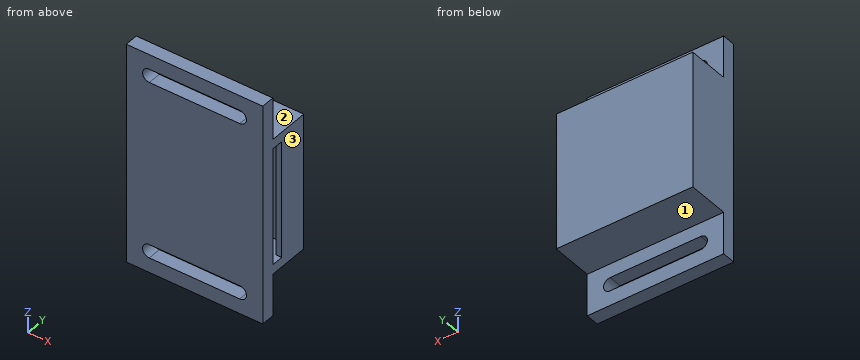
Autodesk Inventor part; units mm, degrees
ref_plane "YZ Plane" through (0, 0, 0) normal (1, 0, 0) x (0, 1, 0)
ref_plane "XZ Plane" through (0, 0, 0) normal (0, 1, 0) x (-1, 0, 0)
ref_plane "XY Plane" through (0, 0, 0) normal (0, 0, 1) x (1, 0, 0)
sketch "Sketch1" plane through (0, 0, 0) normal (0, 1, 0) x (-1, 0, 0)
  line L0 (15.25, -24.65) -> (-15.25, -24.65)
  line L1 (-15.25, -24.65) -> (-15.25, 24.65)
  line L2 (-15.25, 24.65) -> (15.25, 24.65)
  line L3 (15.25, 24.65) -> (15.25, -24.65)
  line L4 (15.25, -24.65) -> (-15.25, 24.65) construction
  line L5 (-15.25, -24.65) -> (15.25, 24.65) construction
  circle A0 centre (10.1, 19.85) radius 1.5
  circle A1 centre (-10.1, 19.85) radius 1.5
  line L6 (10.1, 21.35) -> (-10.1, 21.35)
  circle A2 centre (10.1, -19.85) radius 1.5
  circle A3 centre (-10.1, -19.85) radius 1.5
  line L7 (10.1, -21.35) -> (-10.1, -21.35)
  line L8 (21.35, 0) -> (-21.35, 0) construction
  line L9 (10.1, -18.35) -> (-10.1, -18.35)
  line L10 (10.1, 18.35) -> (-10.1, 18.35)
  line L11 (15.25, -15.25) -> (-15.25, -15.25)
  line L12 (-15.25, -15.25) -> (-15.25, 15.25)
  line L13 (-15.25, 15.25) -> (15.25, 15.25)
  line L14 (15.25, 15.25) -> (15.25, -15.25)
  line L15 (15.25, -15.25) -> (-15.25, 15.25) construction
  line L16 (-15.25, -15.25) -> (15.25, 15.25) construction
  line L17 (0, -34.51) -> (0, 34.51)
  point P0 (0, 0)
  dimension "d11" = 49.3
  dimension "d12" = 30.5
  dimension "d13" = 23.2
  dimension "d14" = 3
  dimension "d15" = 3.3
  dimension "d16" = 30.5
extrude "Extrusion1" add sketch "Sketch1" along normal blind 3 contours L0 L17 L7 A2 L9 L11 L3 | L0 L1 L11 L17 L9 A3 L7 | L11 L17 L13 L3 | L13 L17 L10 A0 L6 L2 L3 | L11 L1 L13 L17 | L13 L1 L2 L17 L6 A1 L10
extrude "Extrusion2" add sketch "Sketch1" along normal blind 12.3 contours L11 L17 L13 L3 | L11 L1 L13 L17
sketch "Sketch2" plane through (0, 12.3, 0) normal (0, 1, 0) x (1, 0, 0)
  line L0 (12.9324, 13.1) -> (-12.9324, 13.1)
  line L1 (-12.9324, 13.1) -> (-12.9324, -13.1)
  line L2 (-12.9324, -13.1) -> (12.9324, -13.1)
  line L3 (12.9324, -13.1) -> (12.9324, 13.1)
  line L4 (12.9324, 13.1) -> (-12.9324, -13.1) construction
  line L5 (-12.9324, 13.1) -> (12.9324, -13.1) construction
  point P0 (0, 0)
  dimension "d21" = 26.2
extrude "Extrusion3" cut sketch "Sketch2" against normal blind 9.3
sketch "Sketch3" plane through (12.9324, 12.3, -13.1) normal (-1, 0, 0) x (0, 0, 1)
  line L0 (26.2, 0) -> (26.2, -9.3)
  line L1 (26.2, -9.3) -> (0, -9.3)
  line L2 (0, 0) -> (0, -9.3)
  line L3 (-2.15, 0) -> (28.35, 0)
  line L4 (0, 0) -> (26.2, 0)
  line L5 (26.2, 0) -> (0, 0)
  line L6 (0, 0) -> (0, -9.3)
  line L7 (0, -9.3) -> (26.2, -9.3)
  line L8 (26.2, -9.3) -> (26.2, 0)
  point P0 (13.1, -12.3)
extrude "Extrusion4" cut sketch "Sketch3" against normal through all
sketch "Sketch6" plane through (0, 12.3, 0) normal (0, 1, 0) x (1, 0, 0)
  line L0 (-15.25, 15.25) -> (-15.25, -15.25)
  line L1 (15.25, 15.25) -> (15.25, 24.65)
  line L2 (-15.25, -15.25) -> (15.25, -15.25)
  line L3 (15.25, -15.25) -> (15.25, 15.25)
  line L4 (15.25, 15.25) -> (-15.25, 15.25)
  line L5 (-15.25, 15.25) -> (-15.25, -15.25)
  point P0 (0, 0)
extrude "Extrusion5" add sketch "Sketch6" against normal blind 3
sketch "Sketch7" plane through (0, 9.3, 0) normal (0, -1, 0) x (1, 0, 0)
  line L0 (15.25, 15.25) -> (15.25, -15.25)
  line L1 (-15.25, 15.25) -> (15.25, 15.25)
  line L2 (15.25, -15.25) -> (13.95, -15.25)
  line L3 (13.95, -15.25) -> (13.95, 15.25)
  line L4 (13.95, 15.25) -> (15.25, 15.25)
  line L5 (15.25, 15.25) -> (15.25, -15.25)
  line L6 (-15.25, -24.65) -> (-15.25, 24.65)
  point P0 (0, 0)
  dimension "d29" = 29.2
extrude "Extrusion6" add sketch "Sketch7" along normal blind 3.6
equation "\"d11\" = length"
equation "\"d12\" = width"
equation "\"d13\" = opening_length"
equation "\"d14\" = opening_width"
equation "\"d15\" = opening_distance_to_edge"
equation "\"d16\" = camera_box_width"
equation "\"d17\" = thickness"
equation "\"d19\" = height"
equation "\"d21\" = inside_width"
equation "\"d22\" = height - thickness"
equation "\"d26\" = thickness"
equation "\"d29\" = inside_width + thickness"
equation "\"d30\" = 1.2 * thickness"
equation "\"width\" = 30.5"
equation "\"length\" = 49.3"
equation "\"opening_width\" = 3"
equation "\"opening_length\" = 23.2"
equation "\"opening_distance_to_edge\" = 3.3"
equation "\"camera_box_width\" = 30.5"
equation "\"thickness\" = 3"
equation "\"inside_width\" = 26.2"
equation "\"height\" = 12.3"
properties part number "bottom" material "SAN Plastic"
The model under review builds one solid part; all positions refer to its coordinate system, in mm. Face numbers are marked on the shaded views. A direction names the side the tool comes from. Coordinates: 2 decimals unless noted, no trailing zeros. Write each loop counter-clockwise with the first axis right and the second up, starting at its lowest first coordinate (ties: lowest second). Pieces come first, ordered by that corner, then holes. Notation, with made-up numbers: (29.25, -23.75) -> (45.25, -23.75) arc R12 ccw to (45.25, -12.75) -> close; hole circle Ø9 at (76, 53). An arc over 180 degrees is marked (long way). Answer in a Markdown table with one row per item.
1. We need section C-C, the plane z = -7. State the section outline as (x, y) points.
Answers below:
| item | result |
|---|---|
| outline | (-15.25, 0) -> (15.25, 0) -> (15.25, 3) -> (-12.93, 3) -> (-12.93, 9.3) -> (13.95, 9.3) -> (13.95, 5.7) -> (15.25, 5.7) -> (15.25, 12.3) -> (-15.25, 12.3) -> close |
2. We need section A-A, the plane x = 3. State the section outline as (y, z) points, and give its area (3 significant figures).
Answers below:
| item | result |
|---|---|
| outline | (0, -24.65) -> (3, -24.65) -> (3, -21.35) -> (0, -21.35) -> close; (0, -18.35) -> (3, -18.35) -> (3, -15.25) -> (12.3, -15.25) -> (12.3, 15.25) -> (3, 15.25) -> (3, 18.35) -> (0, 18.35) -> close; (0, 21.35) -> (3, 21.35) -> (3, 24.65) -> (0, 24.65) -> close; hole (3, -13.1) -> (9.3, -13.1) -> (9.3, 13.1) -> (3, 13.1) -> close |
| area | 248 mm^2 |
3. We need section B-B, the plane y = 4. State the section outline as (x, z) points, and give its area (3 significant figures).
Answers below:
| item | result |
|---|---|
| outline | (-15.25, -15.25) -> (15.25, -15.25) -> (15.25, -13.1) -> (-12.93, -13.1) -> (-12.93, 13.1) -> (15.25, 13.1) -> (15.25, 15.25) -> (-15.25, 15.25) -> close |
| area | 192 mm^2 |
4. For the marked faces 1, 2 and 3, list the 3-axis set-ups (+Z, -Z, +X, -X, +Y, -Y) from which the entire face can be reached by the end or side of a thin tool; tool diameter is ignored.
Answers below:
| item | result |
|---|---|
| face 1 | -Z, +X, -X, +Y |
| face 2 | +Z, +X, -X, +Y |
| face 3 | +Z, -Z, +X, +Y, -Y |
5. Wall thickness on probe 1 along Z at (x, y) = (-7.5, 2.25); probe 2 along Y at (x, z) = (9, 2); probe 3 along Z at (x, y) = (6, 4): over which ranges is each line inside the solid? List them lowest first. Write a range as [from, to].
Answers below:
| item | result |
|---|---|
| probe 1 | z = [-24.65, -21.35], [-18.35, 18.35], [21.35, 24.65] |
| probe 2 | y = [0, 3], [9.3, 12.3] |
| probe 3 | z = [-15.25, -13.1], [13.1, 15.25] |
6. We need section D-D, the plane y = 8. State the section outline as (x, z) points, and give its area (3 significant figures).
Answers below:
| item | result |
|---|---|
| outline | (-15.25, -15.25) -> (15.25, -15.25) -> (15.25, 15.25) -> (-15.25, 15.25) -> close; hole (-12.93, -13.1) -> (13.95, -13.1) -> (13.95, 13.1) -> (-12.93, 13.1) -> close |
| area | 226 mm^2 |
7. Clearance check with flat-ended pins moving along their axes: pin 1 Ø4.5 at (x, y) = (6.5, 5.5) entering from -Z; pin 2 Ø1.9 at (x, y) = (-1, 7) entering from +Z; pin 3 Ø7.5 at (x, z) = (-4, 19.5) entering from +Y. State where each tip first meets the part, or that it passes through.
Answers below:
| item | result |
|---|---|
| pin 1 | stops at z = -15.25 |
| pin 2 | stops at z = 15.25 |
| pin 3 | stops at y = 3 |
